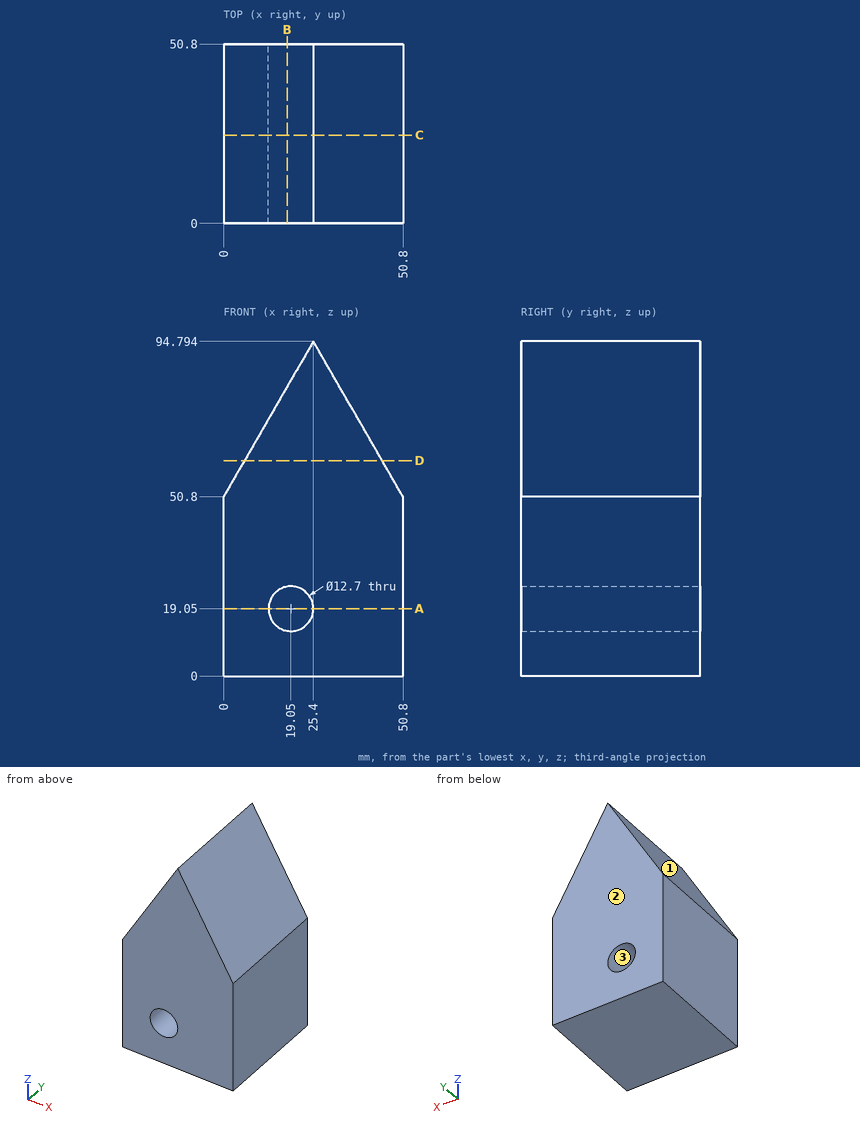
Here's the drawing with two shaded views (mm, measured from the low corner). I have some questions. Give positions to 0.01 mm unless a question says otherwise; leave off trailing zeros. Loops run counter-clockwise (first coordinate to the right, second up) from the corner with the lowest first, then second, coordinate; pieces in that order, holes last. Notation, with made-up numbers: (0, 15) -> (46, 15) arc R13 ccw to (46, 37) -> close; hole circle Ø2 at (54.5, 74.5). An arc over 180 degrees is marked (long way). Use one line per item in the form item = value.
1) If we section it at B-B (x = 18): Please give me the cut outline in (y, z), plus the area to 3 significant figures.
Answers:
outline = (0, 0) -> (50.8, 0) -> (50.8, 12.79) -> (0, 12.79) -> close; (0, 25.31) -> (50.8, 25.31) -> (50.8, 81.98) -> (0, 81.98) -> close
area = 3,530 mm²
2) Will these pins go through, and if not, where does the flat tip stop? pin 1 (4 mm diameter, centred on y = 41, z = 58, fed in from +X); pin 2 (11.5 mm diameter, centred on x = 19.05, z = 19.05, fed in from +Y).
Answers:
pin_1 = 47.8
pin_2 = through
3) I need wall thicknesses on line 1 along X through (y, z) = (35, 19); line 2 along Z through (x, y) = (19.05, 20) (1 decimal); line 3 along Z through (x, y) = (19, 26). Which ranges of each line are inside material? Lowest first, please.
Answers:
line_1 = 0 to 12.7, 25.4 to 50.8
line_2 = 0 to 12.7, 25.4 to 83.8
line_3 = 0 to 12.7, 25.4 to 83.71
4) If we section it at A-A (z = 19.05): Please give me the cut outline in (x, y), plus the area to 3 significant figures.
Answers:
outline = (0, 0) -> (12.7, 0) -> (12.7, 50.8) -> (0, 50.8) -> close; (25.4, 0) -> (50.8, 0) -> (50.8, 50.8) -> (25.4, 50.8) -> close
area = 1,940 mm²
5) We'd pull the mould along Z, two halves only. Please class the marked faces 1, 2 and 3: released by +Z, released by -Z, zero draft, split by the parting line, or undercut.
Answers:
face_1 = released by +Z
face_2 = zero draft
face_3 = undercut
6) If we section it at D-D (z = 61): Please give me the cut outline in (x, y), plus the area to 3 significant figures.
Answers:
outline = (5.89, 0) -> (44.91, 0) -> (44.91, 50.8) -> (5.89, 50.8) -> close
area = 1,980 mm²
7) If we section it at C-C (y = 25): Please give me the cut outline in (x, z).
Answers:
outline = (0, 0) -> (50.8, 0) -> (50.8, 50.8) -> (25.4, 94.79) -> (0, 50.8) -> close; hole circle Ø12.7 at (19.05, 19.05)
